Geometry check sheet. Reference: the model listing, model coordinates, mm. A direction names the side the tool comes from. Give positions to 0.01 mm unless a question says otherwise; leave off trailing zeros. Loops run counter-clockwise (first coordinate to the right, second up) from the corner with the lowest first, then second, coordinate; pieces in that order, holes last. Notation, with made-up numbers: (8.25, -2) - (57.25, -2) arc R16 cw to (57.25, 18) - close; hole circle Ø8 at (22.25, 72). An arc over 180 degrees is marked (long way). Use a Markdown table: item, result. Add a question column.
1. Set-up check for faces 1 (the cylindrical face through (-136.61, 4.54, -14.61)), 2 (the flat face through (-130.175, -6.5, -25)), 3 (the flat face through (136, -6.35, -25)), 4 (the cylindrical face through (-136.61, 4.54, -36.19)): record each of +Z, -Z, +X, -X, +Y, -Y from which the full face is reachable in a straight line by a thin tool's end or side.
2. Cross-section at A-A on z = -26. Enter the section's corners in (x, y) (3 decimals).
3. Material ranges on L1, parallel to X at y = -7.75, z = -37 (3 decimals); L2, parallel to Z at x = 131.5, y = 3.5, recorded low to high.
4. Depth check by flat-ended pin: P1, Ø4, axis at x = 139.5, z = -25.5, coming from the -Y side; P2, Ø6.5, axis at x = -135, z = -24, coming from the +Y side. Enter the tip coordinate at first touch or a pass-through.
5. Cross-section at B-B on z = -42. Enter the section's corners in (x, y) (3 decimals).
from build123d import *

# Parameters (mm, degrees)
F0_W     = 260.35
F0_H     = 19.05
F1_DEPTH = 50.8
F2_W     = 12.7
F2_H     = 25.4
F3_DEPTH = 12.7
F4_R     = 6.34999
F5_W     = 12.7
F5_H     = 25.4
F6_DEPTH = 12.7
F7_R     = 6.34999


# Not quite as in the source:
# - a fillet or chamfer is up to 0.001 mm smaller than in the source, because OpenCascade refuses the exact size


with BuildPart() as f1:
    # F0 (on Top) → F1 (new body)
    with BuildSketch(Plane.XY):
        Rectangle(F0_W, F0_H)
    extrude(amount=-F1_DEPTH)

    # F2 (on face) → F3 (join)
    with BuildSketch(Plane(origin=(-130.175, 0, 0), x_dir=(0, -1, 0), z_dir=(-1, 0, 0))):
        with Locations((0, -25.4)):
            Rectangle(F2_W, F2_H)
    extrude(amount=F3_DEPTH)

    # F4 (radius 6.35 in the source; OpenCascade refuses exactly that, so slightly less here)
    f4_edges = [f1.edges().sort_by_distance(p)[0] for p in [
        (-136.525, 6.35, -12.7),
        (-136.525, -6.35, -12.7),
        (-136.525, -6.35, -38.1),
        (-136.525, 6.35, -38.1),
    ]]
    fillet(f4_edges, radius=F4_R)

    # F5 (on face) → F6 (join)
    with BuildSketch(Plane.YZ.offset(130.175)):
        with Locations((0, -25.4)):
            Rectangle(F5_W, F5_H)
    extrude(amount=F6_DEPTH)

    # F7 (radius 6.35 in the source; OpenCascade refuses exactly that, so slightly less here)
    f7_edges = [f1.edges().sort_by_distance(p)[0] for p in [
        (136.525, -6.35, -12.7),
        (136.525, 6.35, -12.7),
        (136.525, 6.35, -38.1),
        (136.525, -6.35, -38.1),
    ]]
    fillet(f7_edges, radius=F7_R)


solid = f1.part
Values found:
| question | item | result |
|---|---|---|
| 1 | face 1 | +Z, -X, +Y |
| 1 | face 2 | -X, -Y |
| 1 | face 3 | +Z, -Z, +X, -Y |
| 1 | face 4 | -Z, -X, +Y |
| 2 | outline | (-142.875, -6.35) - (-130.175, -6.35) - (-130.175, -9.525) - (130.175, -9.525) - (130.175, -6.35) - (142.875, -6.35) - (142.875, 6.35) - (130.175, 6.35) - (130.175, 9.525) - (-130.175, 9.525) - (-130.175, 6.35) - (-142.875, 6.35) - close |
| 3 | L1 | x = -130.175 to 130.175 |
| 3 | L2 | z = -37.05 to -13.75 |
| 4 | P1 | stops at y = -6.35 |
| 4 | P2 | stops at y = 6.35 |
| 5 | outline | (-130.175, -9.525) - (130.175, -9.525) - (130.175, 9.525) - (-130.175, 9.525) - close |
